Source: CAD feature listing. Evaluate the final solid. Frame: model axes, mm. Face numbers are marked on the shaded views. A direction names the side the tool comes from. Give positions to 0.01 mm unless a question says otherwise; leave off trailing zeros. Loops run counter-clockwise (first coordinate to the right, second up) from the corner with the lowest first, then second, coordinate; pieces in that order, holes last.
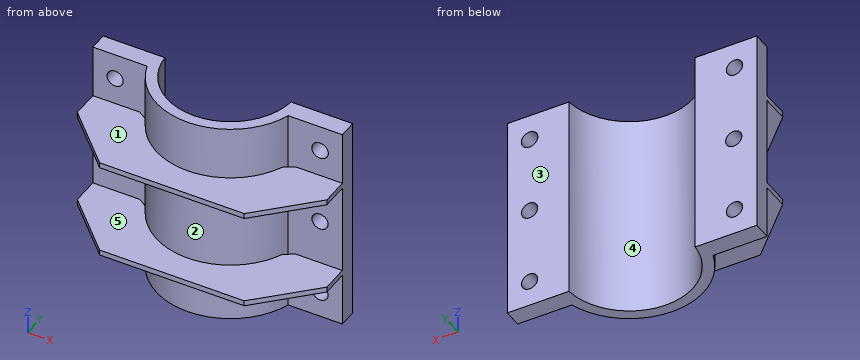
```python
from build123d import *

# Parameters (mm, degrees)
EXTRUDE002_DEPTH         = 6
SKETCH003_R              = 9
SKETCH003_R_2            = 9.18475
EXTRUDE003_DEPTH         = 30
EXTRUDE001_DEPTH         = 115
CLONE002_PLACEMENT_ANGLE = 180


with BuildPart() as extrude002:
    # Sketch002 → Extrude002 (new body)
    with BuildSketch(Plane.XY):
        with BuildLine():
            Line((-138.096095, -175), (-138.096095, -145))
            Line((-138.096095, -145), (-80, -86.903905))
            Line((-80, -86.903905), (80, -86.903905))
            Line((80, -86.903905), (138.096095, -145))
            Line((138.096095, -145), (138.096095, -175))
            Line((138.096095, -175), (86.096095, -175))
            Line((86.096095, -175), (74.344944, -167.222083))
            ThreePointArc((74.344944, -167.222083), (0, -118.75), (-74.344944, -167.222083))
            Line((-86.096095, -175), (-74.344944, -167.222083))
            Line((-138.096095, -175), (-86.096095, -175))
        make_face()
    extrude(amount=EXTRUDE002_DEPTH)


with BuildPart() as extrude002_1:
    # Extrude002 placement: moved
    add(extrude002.part.moved(Location((0, 0, 50))))


with BuildPart() as loch:
    # Sketch003 (on Face3 of Extrude001) → Extrude003 (new body, symmetric)
    with BuildSketch(Plane(origin=(0, -175, 0), x_dir=(-1, 0, 0), z_dir=(0, 1, 0))):
        with Locations((-113.412567, 86.219978)):
            Circle(SKETCH003_R)
        with Locations((-113.412567, -86.219978)):
            Circle(SKETCH003_R_2)
        with Locations((113.412567, -86.219978)):
            Circle(SKETCH003_R)
        with Locations((113.412567, 86.219978)):
            Circle(SKETCH003_R)
        with Locations((112.569069, 0)):
            Circle(SKETCH003_R)
        with Locations((-113.412567, 0)):
            Circle(SKETCH003_R)
    extrude(amount=EXTRUDE003_DEPTH, both=True)


with BuildPart() as cut:
    # Sketch001 → Extrude001 (new body, symmetric)
    with BuildSketch(Plane.XY):
        with BuildLine():
            ThreePointArc((78.096095, -175), (0, -118), (-78.096095, -175))
            Line((-78.096095, -175), (-138.096095, -175))
            Line((-138.096095, -175), (-138.096095, -195))
            Line((-138.096095, -195), (-69.8212, -195))
            ThreePointArc((69.8212, -195), (0, -130), (-69.8212, -195))
            Line((69.8212, -195), (138.096095, -195))
            Line((138.096095, -195), (138.096095, -175))
            Line((138.096095, -175), (78.096095, -175))
        make_face()
    extrude(amount=EXTRUDE001_DEPTH, both=True)

    # Cut: cut Loch
    add(loch.part, mode=Mode.SUBTRACT)


with BuildPart() as obj1:
    # Clone001 base: copy of Extrude002
    add(extrude002_1.part)


with BuildPart() as obj1_1:
    # Clone001 placement: moved
    add(obj1.part.moved(Location((0, 0, -106))))

    # Fusion: union Extrude002, Cut
    add(extrude002_1.part)
    add(cut.part)


with BuildPart() as obj1_2:
    # Clone002 placement: moved
    add(obj1_1.part.moved(Location((0, -400, 0))).rotate(Axis((0, -400, 0), (1, 0, 0)), CLONE002_PLACEMENT_ANGLE))


solid = obj1_2.part
```
(1) Mould query, pull axis Z, two halves, no side actions, for the marked faces 1, 2 and 3. Classes: pulls with the +Z half, pulls with the -Z half, needs draft (parallel to the pull), parting line crosses it, or undercut.
A:
face 1: pulls with the +Z half
face 2: undercut
face 3: needs draft
(2) Section A-A, the plane z = 0. Return the cut outline in (x, y), then the cut area to 3 significant figures.
A:
outline: (-138.1, -225) - (-121.57, -225) - (-121.57, -205) - (-138.1, -205) - close; (-103.57, -225) - (-78.1, -225) arc R82 ccw to (78.1, -225) - (104.41, -225) - (104.41, -205) - (69.82, -205) arc R70 cw to (-69.82, -205) - (-103.57, -205) - close; (122.41, -225) - (138.1, -225) - (138.1, -205) - (122.41, -205) - close
area: 4,330 mm2
(3) Reachability of the marked faces 4 and 5 from +Z, -Z, +X, -X, +Y, -Y: full face, straight path, thin tool, end or side. Return the list, or none.
A:
face 4: +Z, -Z, +Y
face 5: -Y
(4) Section C-C, the plane x = -116. Return the cut outline in (y, z).
A:
outline: (-277.1, -56) - (-225, -56) - (-225, -77.6) - (-205, -77.6) - (-205, -8.32) - (-225, -8.32) - (-225, -50) - (-277.1, -50) - close; (-277.1, 50) - (-225, 50) - (-225, 8.32) - (-205, 8.32) - (-205, 77.6) - (-225, 77.6) - (-225, 56) - (-277.1, 56) - close; (-225, -115) - (-205, -115) - (-205, -94.84) - (-225, -94.84) - close; (-225, 94.84) - (-205, 94.84) - (-205, 115) - (-225, 115) - close
(5) Ray query, line 1 along X through (y, z) = (-219.75, 0); line 2 along Z through (x, y) = (-98, -266); line 3 along Z through (x, y) = (-114, -219.5). Return the intervals inside material, ascending.
A:
line 1: x = -138.1 to -121.57, -103.57 to -67.16, 67.16 to 104.41, 122.41 to 138.1
line 2: z = -56 to -50, 50 to 56
line 3: z = -115 to -95.2, -77.24 to -8.89, 8.89 to 77.24, 95.2 to 115
(6) Section D-D, the plane x = 35.5. Return the cut outline in (y, z), then the cut area to 3 significant figures.
A:
outline: (-313.1, -56) - (-273.92, -56) - (-273.92, -115) - (-260.33, -115) - (-260.33, 115) - (-273.92, 115) - (-273.92, 56) - (-313.1, 56) - (-313.1, 50) - (-273.92, 50) - (-273.92, -50) - (-313.1, -50) - close
area: 3,600 mm2
(7) First-contact query: pin 1 (8 mm diameter, centred on x = -68.5, z = 35.5, fed in from -Y); pin 2 (21 mm diameter, centred on x = 113.41, z = 86.22, fed in from -Y); pin 3 (3 mm diameter, centred on x = 46.5, y = -278, fed in from -Z); pin 4 (20.5 mm diameter, centred on x = -113.41, z = -86.22, fed in from +Y). Flat tips, straight axial feed; report the tip coordinate or a pass-through.
A:
pin 1: stops at y = -250.63
pin 2: stops at y = -225
pin 3: stops at z = -56
pin 4: stops at y = -205
(8) Section B-B, the plane y = -301. Return the cut outline in (x, z), then the cut area to 3 significant figures.
A:
outline: (-92.1, -56) - (92.1, -56) - (92.1, -50) - (-92.1, -50) - close; (-92.1, 50) - (92.1, 50) - (92.1, 56) - (-92.1, 56) - close
area: 2,210 mm2
